Read the model definition and answer for the solid it produces. Units are mm, in the model's axes. Face numbers are marked on the shaded views. A direction names the side the tool comes from. Give positions to 0.01 mm unless a question says otherwise; leave off trailing zeros. Write each loop counter-clockwise with the first axis right and the second up, starting at its lowest first coordinate (ties: lowest second). Pieces come first, ordered by that corner, then holes. Notation, with made-up numbers: M 54.5,89 L 85.5,89 A15 cw 85.5,116 Z; hole C 2.25,20.25 d1. An arc over 180 degrees is marked long. Put each result on its own line as item: value.
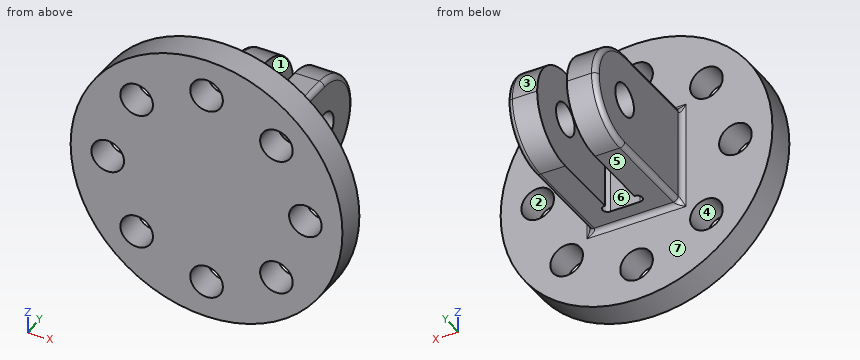
Autodesk Inventor part; units mm, degrees
ref_plane "YZ Plane" through (0, 0, 0) normal (1, 0, 0) x (0, 1, 0)
ref_plane "XZ Plane" through (0, 0, 0) normal (0, 1, 0) x (-1, 0, 0)
ref_plane "XY Plane" through (0, 0, 0) normal (0, 0, 1) x (1, 0, 0)
sketch "Sketch1" plane through (0, 0, 0) normal (0, 1, 0) x (-1, 0, 0)
  circle A0 centre (0, 0) radius 27.5
  dimension "d0" = 55
extrude "Extrusion1" add sketch "Sketch1" along normal blind 6
sketch "Sketch2" plane through (0, 6, 0) normal (0, 1, 0) x (1, 0, 0)
  circle A0 centre (0, 0) radius 27.5
  point P0 (20, 0)
  point P1 (14.1421, 14.1421)
  point P2 (0, 20)
  point P3 (-14.1421, 14.1421)
  point P4 (-20, 0)
  point P5 (-14.1421, -14.1421)
  point P6 (0, -20)
  point P7 (14.1421, -14.1421)
  dimension "d3" = 20
  dimension "d6" = 360
hole "Hole1" at (20, 6, 0) at (14.1421, 6, -14.1421) at (0, 6, -20) at (-14.1421, 6, -14.1421) at (-20, 6, 0) at (-14.1421, 6, 14.1421) at (0, 6, 20) at (14.1421, 6, 14.1421) direction (0, -1, 0) diameter 6.6 depth 8 tip angle 118
sketch "Sketch8" plane through (0, 6, 0) normal (0, 1, 0) x (1, 0, 0)
  circle A0 centre (0, 0) radius 27.5
  line L0 (-9, 10) -> (9, 10)
  line L1 (9, 10) -> (9, -10)
  line L2 (9, -10) -> (-9, -10)
  line L3 (-9, -10) -> (-9, 10)
  point P0 (0, 10)
  point P1 (9, 0)
  dimension "d28" = 18
  dimension "d30" = 20
extrude "Extrusion3" add sketch "Sketch8" along normal blind 30 contours L0 L1 L2 L3
sketch "Sketch9" plane through (0, 36, 0) normal (0, 1, 0) x (1, 0, 0)
  line L0 (9, 10) -> (-9, 10)
  line L1 (-9, -10) -> (9, -10)
  line L2 (-3, 10) -> (3, 10)
  line L3 (3, 10) -> (3, -10)
  line L4 (3, -10) -> (-3, -10)
  line L5 (-3, -10) -> (-3, 10)
  point P0 (0, 0)
  point P1 (0, 10)
  point P2 (0, 10)
  dimension "d54" = 6
sketch "Sketch10" plane through (9, 6, 10) normal (1, 0, 0) x (0, 0, -1)
  line L0 (20, 0) -> (0, 0)
  line L1 (20, 0) -> (20, 30)
  line L2 (0, 30) -> (20, 30)
  line L3 (0, 0) -> (0, 30)
  point P0 (10, -6)
fillet "Fillet2" radius 10 2 edges at (0, 36, 10) (0, 36, -10)
sketch "Sketch11" plane through (9, 6, 10) normal (1, 0, 0) x (0, 0, -1)
  arc A0 (20, 20) -> (0, 20) centre (10, 20) ccw
  point P0 (10, -6)
hole "Hole3" at (9, 26, 0) direction (-1, 0, 0) diameter 6.6 end through all
extrude "Extrusion4" cut sketch "Sketch9" against normal blind 25
sketch "Sketch12" plane through (-9, 6, 10) normal (0, 0, 1) x (1, 0, 0)
  line L0 (6, 5) -> (6, 20)
  line L1 (12, 20) -> (12, 5)
  line L2 (12, 5) -> (6, 5)
  arc A0 (6, 6) -> (6, 4) centre (6, 5) ccw
  line L3 (6, 5) -> (6, 4) construction
  line L4 (6, 5) -> (6, 6) construction
  arc A1 (12, 4) -> (12, 6) centre (12, 5) ccw
  line L5 (12, 5) -> (12, 4) construction
  line L6 (12, 5) -> (12, 6) construction
  line L7 (6, 6) -> (12, 6)
  line L8 (6, 4) -> (12, 4)
  point P0 (9, -6)
  dimension "d45" = 1
  dimension "d46" = 180
  dimension "d47" = 1
  dimension "d48" = 180
extrude "Extrusion5" cut sketch "Sketch12" against normal through all contours L2 L1 A1 L8 A0 L0
fillet "Fillet3" radius 1 4 edges at (0, 6, 10) (-9, 6, 0) (9, 6, 0) (0, 6, -10)
fillet "Fillet4" radius 1 10 edges at (9, 33.0711, -7.0711) (9, 16.5001, -10) (9.2929, 6.2929, -10.2929) (9.2929, 6.2929, 10.2929) (9, 16.5001, 10) (-9, 33.0711, -7.0711) (-9, 16.5001, 10) (-9.2929, 6.2929, 10.2929) (-9.2929, 6.2929, -10.2929) (-9, 16.5001, -10)
properties part number "right_angle_holder"
(1) Given pin 1 Ø8 at (x, z) = (14, -10.5) entering from +Y; pin 2 Ø1 at (x, z) = (-2.5, -15.5) entering from -Y; pin 3 Ø6 at (y, z) = (22, -2.5) entering from -X; pin 4 Ø1 at (y, z) = (16.5, -7) entering from +X, each flat-ended and moving along its own axis, determine where each tip first touches the part or whether it passes through.
Result:
pin 1: stops at y = 6
pin 2: stops at y = 0
pin 3: stops at x = -9
pin 4: stops at x = 9
(2) Section A-A on x = 0 is taken. Determine the outline of the cut face in (y, z).
Result:
outline: M 0,-27.5 L 6,-27.5 L 6,-23.3 L 0,-23.3 Z; M 0,-16.7 L 6,-16.7 L 6,-11 A1 cw 7,-10 L 10,-10 L 10,10 L 7,10 A1 cw 6,11 L 6,16.7 L 0,16.7 Z; M 0,23.3 L 6,23.3 L 6,27.5 L 0,27.5 Z
(3) Section D-D on x = 20 is taken. Determine the outline of the cut face in (y, z), and give its area (3 significant figures).
Result:
outline: M 0,-18.87 L 6,-18.87 L 6,-3.3 L 0,-3.3 Z; M 0,3.3 L 6,3.3 L 6,18.87 L 0,18.87 Z
area: 187 mm²
(4) For a pull along Z with two mould halves and no side action, classify the marked faces 1, 2, 3 and 4 as +Z half, -Z half, draft (parallel to the pull), parting line (faces both ways), or undercut.
Result:
face 1: draft
face 2: undercut
face 3: +Z half
face 4: undercut
(5) Section C-C on z = -20 is taken. Determine the outline of the cut face in (x, y), and give its area (3 significant figures).
Result:
outline: M -18.87,0 L -3.3,0 L -3.3,6 L -18.87,6 Z; M 3.3,0 L 18.87,0 L 18.87,6 L 3.3,6 Z
area: 187 mm²
(6) Which of the six approach directions +Z, -Z, +X, -X, +Y, -Y give full straight-line access (tool end or side, diameter ignored) to the marked faces 5, 6 and 7?
Result:
face 5: -Z, +X, -X, +Y
face 6: +Z, -Z, +Y
face 7: +Y
(7) Straight lines are drawn through the part: line 1 along Z through (x, y) = (0, 4); line 2 along X through (y, z) = (4.5, -13); line 3 along X through (y, z) = (18, -2.5). For each, find the intervals that lie inside material, in ascending order. Write a range as from..to.
Result:
line 1: z = -27.5..-23.3, -16.7..16.7, 23.3..27.5
line 2: x = -24.23..-17.24, -11.05..11.05, 17.24..24.23
line 3: x = -9..-3, 3..9
(8) Section B-B on z = -14.5 is taken. Determine the outline of the cut face in (x, y).
Result:
outline: M -23.37,0 L -17.42,0 L -17.42,6 L -23.37,6 Z; M -10.86,0 L 10.86,0 L 10.86,6 L -10.86,6 Z; M 17.42,0 L 23.37,0 L 23.37,6 L 17.42,6 Z
